```python
from build123d import *

# Parameters (mm, degrees)
F0_W     = 25.4
F0_H     = 25.4
F1_DEPTH = 12.7
F3_DEPTH = 12.7
F4_R     = 26.692989
F4_R_2   = 12.7
F5_DEPTH = 12.7


with BuildPart() as f1:
    # F0 (on Top) → F1 (new body, symmetric)
    with BuildSketch(Plane.XY):
        Rectangle(F0_W, F0_H)
    extrude(amount=F1_DEPTH, both=True)

    # F2 (on Front) → F3 (cut, symmetric)
    with BuildSketch(Plane.XZ):
        Polygon((-12.7, -12.7), (0, 12.7), (12.7, -12.7), (26.629834, -12.7), (26.629834, 23.978902), (-32.895677, 23.978902), (-32.895677, -12.7), align=None)
    extrude(amount=F3_DEPTH, both=True, mode=Mode.SUBTRACT)

    # F4 (on Top) → F5 (cut, symmetric)
    with BuildSketch(Plane.XY):
        Circle(F4_R)
        Circle(F4_R_2, mode=Mode.SUBTRACT)
    extrude(amount=F5_DEPTH, both=True, mode=Mode.SUBTRACT)


solid = f1.part
```
Part model, mm, in its own coordinate system. Coordinates: 2 decimals unless noted, no trailing zeros. Order: outer loops, then holes, each group sorted by start corner. A loop starts at its lowest first (then second) coordinate and runs counter-clockwise, first axis right, second up. Notation, with made-up numbers: (9, -22.5) - (56, -22.5) arc R25 ccw to (56, 12.5) - close; hole circle Ø2 at (53.5, 69). An arc over 180 degrees is marked (long way). Return JSON: item names as keys, results as strings. Group by question number.
Item 1: Pin check, flat tips, straight feed: pin 1 (5 mm diameter, centred on y = 8.5, z = -5, fed in from -X); pin 2 (4 mm diameter, centred on x = 2.5, y = -5, fed in from +Z); pin 3 (2 mm diameter, centred on y = 6, z = -5, fed in from +X). Stop position of each tip, or through.
Item 2: Cut at C-C (z = 6.5). List the corners of the cut face in (x, y).
Item 3: Cut at B-B (x = -8.75). List the corners of the cut face in (y, z), plus the area to 3 significant figures.
Item 4: Drill centre lines: probe 1 along Z at (x, y) = (-9.75, -3); probe 2 along Z at (x, y) = (-6, 8.25); probe 3 along X at (y, z) = (-10.75, 7.25) (3 decimals). Where is each one in solid material? Low to high. Write a range as from..to.
Item 5: Cut at A-A (y = 7.25). List the corners of the cut face in (x, z), plus the area to 3 significant figures.
Item 6: Cut at D-D (y = -1.5). List the corners of the cut face in (x, z), plus the area to 3 significant figures.
Check values:
{
 "1": {"pin 1": "stops at x = -10.05", "pin 2": "stops at z = 11.7", "pin 3": "stops at x = 9.35"},
 "2": {"outline": "(-3.1, -12.32) arc R12.7 ccw to (3.1, -12.32) - (3.1, 12.32) arc R12.7 ccw to (-3.1, 12.32) - close"},
 "3": {"outline": "(-9.2, -12.7) - (9.2, -12.7) - (9.2, -4.8) - (-9.2, -4.8) - close", "area": "145 mm2"},
 "4": {"probe 1": "z = -12.7..-6.8", "probe 2": "z = -12.7..0.7", "probe 3": "x = -2.725..2.725"},
 "5": {"outline": "(-10.43, -12.7) - (10.43, -12.7) - (10.43, -8.15) - (0, 12.7) - (-10.43, -8.15) - close", "area": "312 mm2"},
 "6": {"outline": "(-12.61, -12.7) - (12.61, -12.7) - (12.61, -12.52) - (0, 12.7) - (-12.61, -12.52) - close", "area": "323 mm2"}
}
